Input: part model. Units: mm. Frame: model coordinates. Face numbers are marked on the shaded views. A direction names the side the tool comes from. Give positions to 0.01 mm unless a question says otherwise; leave off trailing zeros. Write each loop counter-clockwise with the first axis right and the second up, starting at its lowest first coordinate (ties: lowest second). Pieces come first, ordered by that corner, then holes.
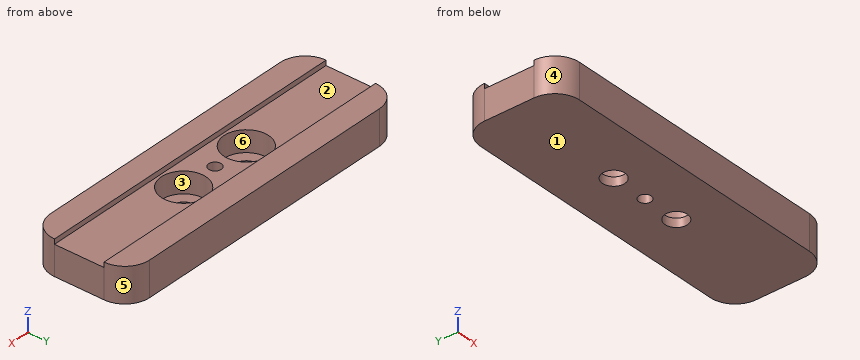
```python
from build123d import *

# Parameters (mm, degrees)
SKETCH_1_W                   = 130
SKETCH_1_H                   = 40
EXTRUDE_1_DEPTH              = 14
HOLE_WIZARD_M6_1_D           = 5
SKETCH_8_W                   = 130
SKETCH_8_H                   = 20
CUT_EXTRUDE_1_DEPTH          = 2
HOLE_WIZARD_M8_1_D           = 9
HOLE_WIZARD_M8_1_CBORE_D     = 18
HOLE_WIZARD_M8_1_CBORE_DEPTH = 8.5
FILLET_1_R                   = 10


with BuildPart() as part:
    # 草图1 → 凸台-拉伸1 (new body)
    with BuildSketch(Plane.XY):
        with Locations((0, 20)):
            Rectangle(SKETCH_1_W, SKETCH_1_H)
    extrude(amount=EXTRUDE_1_DEPTH)

    # M6 螺纹孔1 (through all)
    with Locations(Plane.XY.offset(14)):
        with Locations((0, 20)):
            Hole(HOLE_WIZARD_M6_1_D / 2)

    # 草图8 → 切除-拉伸1 (cut)
    with BuildSketch(Plane.XY.offset(14)):
        with Locations((0, 20)):
            Rectangle(SKETCH_8_W, SKETCH_8_H)
    extrude(amount=-CUT_EXTRUDE_1_DEPTH, mode=Mode.SUBTRACT)

    # M8 六角头螺栓的柱形沉头孔1 (through all)
    with Locations(Plane.XY.offset(12)):
        with Locations((-15, 20), (15, 20)):
            CounterBoreHole(HOLE_WIZARD_M8_1_D / 2, HOLE_WIZARD_M8_1_CBORE_D / 2, HOLE_WIZARD_M8_1_CBORE_DEPTH)

    # 圆角1
    fillet_1_edges = [part.edges().sort_by_distance(p)[0] for p in [
        (65, 0, 7),
        (65, 40, 7),
        (-65, 0, 7),
        (-65, 40, 7),
    ]]
    fillet(fillet_1_edges, radius=FILLET_1_R - 0.0001)  # a hair under: the kernel refuses the full size


solid = part.part
```
Item 1: Section A-A (x = -15). Return loops of the section in (y, z), and give its area (4 significant figures).
Item 2: Set-up query: the marked faces 1 and 2. Return all of +Z, -Z, +X, -X, +Y, -Y with unobstructed straight access to the full face (end or side cutting, diameter ignored); none if empty.
Item 3: Section C-C (y = 20). Return loops of the section in (x, z).
Item 4: Mould query, pull axis X, two halves, no side actions, for the marked faces 3, 4, 5 and 6. Classes: +X half, -X half, draft (parallel to the pull), parting line (faces both ways), or undercut.
Item 5: Section D-D (x = -35.5). Return loops of the section in (y, z), and give its area (3 significant figures).
Item 6: Ray query, line 1 (Y direction, x = 0, z = 8.75); line 2 (Y direction, x = 15, z = 10); line 3 (X direction, y = 14.5, z = 4). Return the intervals inside material, ascending.
Item 7: Section B-B (z = 10). Return loops of the section in (x, y), and give its area (3 significant figures).
Item 8: Pin query (flat end, axial travel): pin 1 (11.5 mm diameter, centred on x = 15, y = 20, fed in from +Z); pin 2 (6 mm diameter, centred on x = 0, y = 20, fed in from +Z); pin 3 (5.5 mm diameter, centred on x = -15, y = 20, fed in from -Z). Return the tip coordinate at first contact, or that it passes through.
Solved:
1. outline: (0, 0) - (15.5, 0) - (15.5, 3.5) - (11, 3.5) - (11, 12) - (10, 12) - (10, 14) - (0, 14) - close; (24.5, 0) - (40, 0) - (40, 14) - (30, 14) - (30, 12) - (29, 12) - (29, 3.5) - (24.5, 3.5) - close
1. area: 335.5 mm2
2. face 1: -Z, +X, -X, +Y, -Y
2. face 2: +Z, +X, -X
3. outline: (-65, 0) - (-19.5, 0) - (-19.5, 3.5) - (-24, 3.5) - (-24, 12) - (-65, 12) - close; (-10.5, 0) - (-2.5, 0) - (-2.5, 12) - (-6, 12) - (-6, 3.5) - (-10.5, 3.5) - close; (2.5, 0) - (10.5, 0) - (10.5, 3.5) - (6, 3.5) - (6, 12) - (2.5, 12) - close; (19.5, 0) - (65, 0) - (65, 12) - (24, 12) - (24, 3.5) - (19.5, 3.5) - close
4. face 3: undercut
4. face 4: -X half
4. face 5: +X half
4. face 6: undercut
5. outline: (0, 0) - (40, 0) - (40, 14) - (30, 14) - (30, 12) - (10, 12) - (10, 14) - (0, 14) - close
5. area: 520 mm2
6. line 1: y = 0 to 17.5, 22.5 to 40
6. line 2: y = 0 to 11, 29 to 40
6. line 3: x = -65 to -22.12, -7.88 to 7.88, 22.12 to 65
7. outline: (-65, 10) arc R10 ccw to (-55, 0) - (55, 0) arc R10 ccw to (65, 10) - (65, 30) arc R10 ccw to (55, 40) - (-55, 40) arc R10 ccw to (-65, 30) - close; hole circle Ø18 at (-15, 20); hole circle Ø5 at (0, 20); hole circle Ø18 at (15, 20)
7. area: 4,590 mm2
8. pin 1: stops at z = 3.5
8. pin 2: stops at z = 12
8. pin 3: passes through
